Here's the drawing with two shaded views (mm, measured from the low corner). I have some questions. Give positions to 0.01 mm unless a question says otherwise; leave off trailing zeros. Loops run counter-clockwise (first coordinate to the right, second up) from the corner with the lowest first, then second, coordinate; pieces in that order, holes last. Notation, with made-up numbers: (88.25, 41.5) - (127.25, 41.5) arc R21 ccw to (127.25, 50.5) - close; hole circle Ø10 at (36.5, 71). An arc over 180 degrees is marked (long way). Write each question's results on one line, items separated by ' | '. Start each with the question number.
1) I want a section at A-A, the plane x = 10. Write out the boundary of the cut face in (y, z), and give its area (3 significant figures).
2) I'm going to push a flat-ended pin straight in: pin 1 (3 mm diameter, centred on x = 34, y = 37.836, fed in from +Z). Where does the tip first touch, or does it pass through?
3) I want a section at B-B, the plane y = 7. Write out the boundary of the cut face in (x, z), and give its area (3 significant figures).
4) If I drill on probe 1 along Y at (x, z) = (10, 6); probe 2 along Y at (x, z) = (35.5, 3.75); probe 3 along X at (y, z) = (8.5, 5.5), over which ranges is the centre line in solid material (lowest first)? Write a range as [from, to].
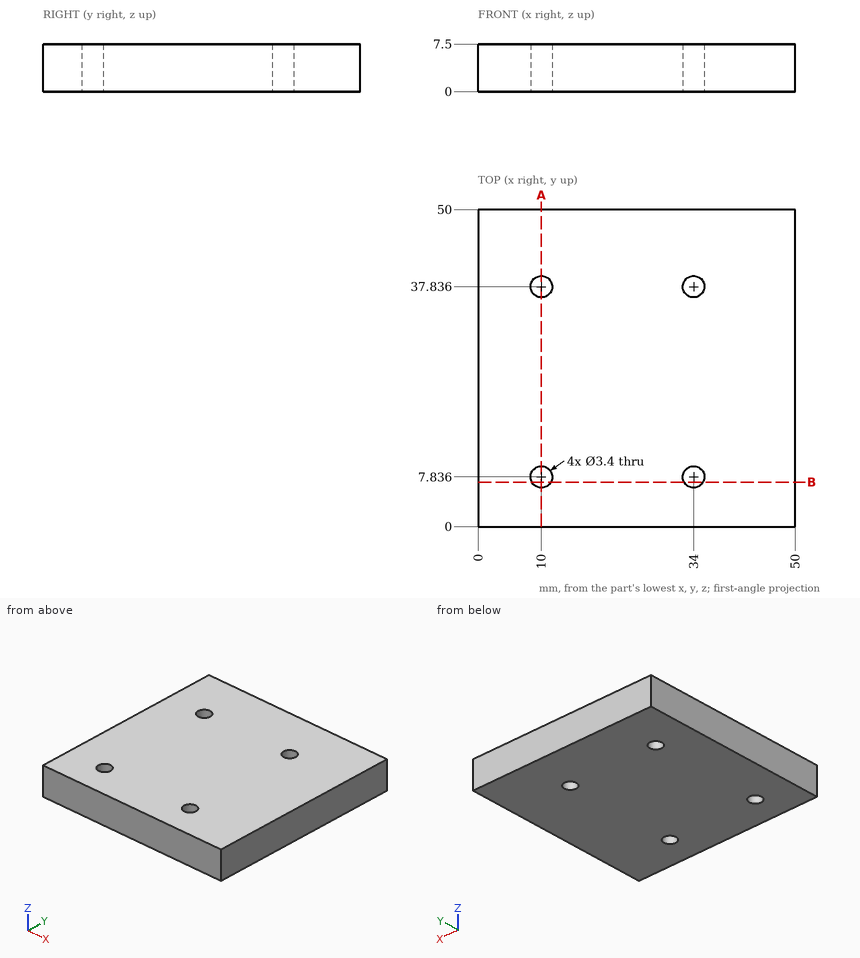
Answers:
1) outline: (0, 0) - (6.14, 0) - (6.14, 7.5) - (0, 7.5) - close; (9.54, 0) - (36.14, 0) - (36.14, 7.5) - (9.54, 7.5) - close; (39.54, 0) - (50, 0) - (50, 7.5) - (39.54, 7.5) - close | area: 324 mm2
2) pin 1: passes through
3) outline: (0, 0) - (8.52, 0) - (8.52, 7.5) - (0, 7.5) - close; (11.48, 0) - (32.52, 0) - (32.52, 7.5) - (11.48, 7.5) - close; (35.48, 0) - (50, 0) - (50, 7.5) - (35.48, 7.5) - close | area: 331 mm2
4) probe 1: y = [0, 6.14], [9.54, 36.14], [39.54, 50] | probe 2: y = [0, 7.04], [8.64, 37.04], [38.64, 50] | probe 3: x = [0, 8.44], [11.56, 32.44], [35.56, 50]
